Autodesk Inventor part; units mm, degrees
ref_plane "YZ Plane" through (0, 0, 0) normal (1, 0, 0) x (0, 1, 0)
ref_plane "XZ Plane" through (0, 0, 0) normal (0, 1, 0) x (-1, 0, 0)
ref_plane "XY Plane" through (0, 0, 0) normal (0, 0, 1) x (1, 0, 0)
sketch "Sketch1" plane through (0, 0, 0) normal (0, 0, 1) x (1, 0, 0)
  line L0 (0, 0) -> (46.0996, 0)
  line L1 (46.0996, 0) -> (46.0996, 41.4402)
  line L2 (46.0996, 41.4402) -> (0, 41.4402)
  line L3 (0, 41.4402) -> (0, 0)
  line L4 (6.0482, 32.1555) -> (39.3637, 32.1555)
  line L5 (39.3637, 32.1555) -> (39.3637, 8.4888)
  line L6 (39.3637, 8.4888) -> (6.0482, 8.4888)
  line L7 (6.0482, 8.4888) -> (6.0482, 32.1555)
extrude "Extrusion1" add sketch "Sketch1" along normal blind 60
fillet "Fillet1" radius 5 1 edges at (23.0498, 0, 60)
chamfer "Chamfer1" distance 2 angle 45 3 edges at (46.0996, 23.2201, 60) (46.0996, 1.4645, 58.5355) (46.0996, 0, 27.5)
properties material "Steel, Alloy"
Verification items for the finished model (mm, model axes). A direction names the side the tool comes from. Round coordinates to 2 decimals unless told otherwise and drop trailing zeros. Order: outer loops, then holes, each group sorted by start corner. A loop starts at its lowest first (then second) coordinate and runs counter-clockwise, first axis right, second up.
1) Cross-section at A-A, the plane y = 14.5. Record the cut outline in (x, z), plus the area to 3 significant figures.
Geometry says:
outline: (0, 0) - (6.05, 0) - (6.05, 60) - (0, 60) - close; (39.36, 0) - (46.1, 0) - (46.1, 58) - (44.1, 60) - (39.36, 60) - close
area: 765 mm2
2) Cross-section at B-B, the plane x = 33. Record the cut outline in (y, z), plus the area to 3 significant figures.
Geometry says:
outline: (0, 0) - (8.49, 0) - (8.49, 60) - (5, 60) arc R5 ccw to (0, 55) - close; (32.16, 0) - (41.44, 0) - (41.44, 60) - (32.16, 60) - close
area: 1,060 mm2
3) Cross-section at C-C, the plane z = 7.5. Record the cut outline in (x, y), plus the area to 3 significant figures.
Geometry says:
outline: (0, 0) - (44.1, 0) - (46.1, 2) - (46.1, 41.44) - (0, 41.44) - close; hole (6.05, 8.49) - (39.36, 8.49) - (39.36, 32.16) - (6.05, 32.16) - close
area: 1,120 mm2
4) Material ranges on line 1 (X direction, y = 15.5, z = 46.5); line 2 (Y direction, x = 23, z = 9.5); line 3 (Y direction, x = 24, z = 56), recorded low to high.
Geometry says:
line 1: x = 0 to 6.05, 39.36 to 46.1
line 2: y = 0 to 8.49, 32.16 to 41.44
line 3: y = 0.1 to 8.49, 32.16 to 41.44
5) Tool access check on faces 4 (the flat face through (39.364, 20, 30)), 5 (the flat face through (45.1, 23, 59)). Record the directions out of +Z, -Z, +X, -X, +Y, -Y that give a thin tool (end or side, any length) a straight path to the whole face; none if there is none.
Geometry says:
face 4: +Z, -Z
face 5: +Z, +X, +Y, -Y
6) Draft check along X on faces 1 (the flat face through (0, 21, 30)), 2 (the flat face through (6.048, 20, 30)), 3 (the cylindrical face through (22, 2, 59)). Enter one of: +X half, -X half, draft (parallel to the pull), parting line (faces both ways), or undercut.
Geometry says:
face 1: -X half
face 2: undercut
face 3: draft
